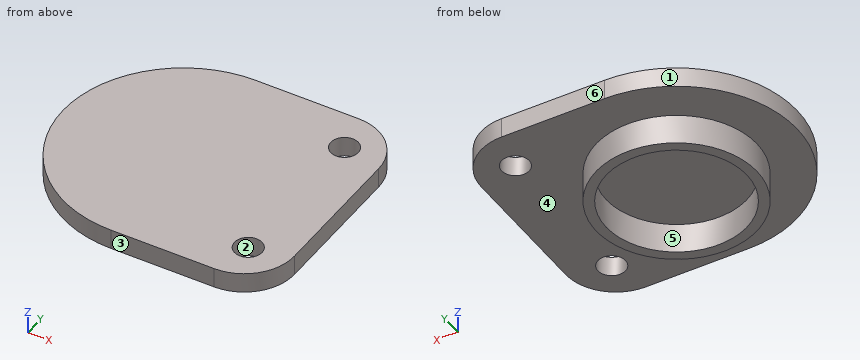
from build123d import *

# Parameters (mm, degrees)
SKETCH1_R           = 2.75
BOSS_EXTRUDE1_DEPTH = 4
SKETCH2_R           = 16
SKETCH2_R_2         = 14
BOSS_EXTRUDE2_DEPTH = 6


with BuildPart() as part:
    # Sketch1 → Boss-Extrude1 (new body)
    with BuildSketch(Plane.XY):
        with BuildLine():
            Line((0, -24), (20.5, -24))
            ThreePointArc((20.5, -24), (27.571067812, -21.071067812), (30.5, -14))
            Line((30.5, -14), (30.5, 14))
            ThreePointArc((30.5, 14), (27.571067812, 21.071067812), (20.5, 24))
            Line((20.5, 24), (0, 24))
            ThreePointArc((0, 24), (-24, 0), (0, -24))
        make_face()
        with Locations((22.5, -16)):
            Circle(SKETCH1_R, mode=Mode.SUBTRACT)
        with Locations((22.5, 16)):
            Circle(SKETCH1_R, mode=Mode.SUBTRACT)
    extrude(amount=BOSS_EXTRUDE1_DEPTH)

    # Sketch2 → Boss-Extrude2 (add)
    with BuildSketch(Plane(origin=(0, 0, 0), x_dir=(-1, 0, 0), z_dir=(0, 0, -1))):
        Circle(SKETCH2_R)
        Circle(SKETCH2_R_2, mode=Mode.SUBTRACT)
    extrude(amount=BOSS_EXTRUDE2_DEPTH)


solid = part.part
The listing builds one solid part. Answer for the finished solid, in the listing's coordinates (mm). Face numbers are marked on the shaded views. A direction names the side the tool comes from. Give positions to 0.01 mm unless a question says otherwise; leave off trailing zeros. Write each loop counter-clockwise with the first axis right and the second up, starting at its lowest first coordinate (ties: lowest second). Pieces come first, ordered by that corner, then holes. Notation, with made-up numbers: (-2, 29.25) -> (45, 29.25) arc R25 cw to (45, 44.25) -> close; hole circle Ø10 at (-7, 57). An arc over 180 degrees is marked (long way). One line per question, with ' | ' between items. Start each with the question number.
1. For a pull along Y with two mould halves and no side action, classify the marked faces 1, 2, 3 and 4 as pulls with the +Y half, pulls with the -Y half, needs draft (parallel to the pull), parting line crosses it, or undercut.
2. Section D-D (y = 0) is taken. Determine the outline of the cut face in (x, z).
3. Section B-B (x = 22.5) is taken. Determine the outline of the cut face in (y, z), plus the area to 3 significant figures.
4. Given pin 1 Ø5 at (y, z) = (-8, -4) entering from -X (3 decimals); pin 2 Ø6 at (x, z) = (-13.5, 1.5) entering from -Y; pin 3 Ø2 at (x, y) = (-17.5, 1) entering from -Z; pin 4 Ø1.5 at (x, z) = (5.5, -0.5) entering from +Y, each flat-ended and moving along its own axis, determine where each tip first touches the part or whether it passes through.
5. Section A-A (z = 0.75) is taken. Determine the outline of the cut face in (x, y), plus the area to 3 significant figures.
6. Find the intervals of material crossed by probe 1 along Y at (x, z) = (22.5, 1.35); probe 2 along Y at (x, z) = (0, -1.4); probe 3 along Z at (x, y) = (-0.5, 12.5), in increasing order.
7. Section C-C (y = -12) is taken. Determine the outline of the cut face in (x, z).
8. For the marked faces 5 and 6, determine the directions among +Z, -Z, +X, -X, +Y, -Y from which every point of the face is accessible in a straight line to the end or side of a thin tool.
Response values:
1) face 1: parting line crosses it | face 2: undercut | face 3: pulls with the -Y half | face 4: needs draft
2) outline: (-24, 0) -> (-16, 0) -> (-16, -6) -> (-14, -6) -> (-14, 0) -> (14, 0) -> (14, -6) -> (16, -6) -> (16, 0) -> (30.5, 0) -> (30.5, 4) -> (-24, 4) -> close
3) outline: (-23.8, 0) -> (-18.75, 0) -> (-18.75, 4) -> (-23.8, 4) -> close; (-13.25, 0) -> (13.25, 0) -> (13.25, 4) -> (-13.25, 4) -> close; (18.75, 0) -> (23.8, 0) -> (23.8, 4) -> (18.75, 4) -> close | area: 146 mm2
4) pin 1: x = -15.025 | pin 2: y = -21.58 | pin 3: z = 0 | pin 4: y = 24
5) outline: (0, -24) -> (20.5, -24) arc R10 ccw to (30.5, -14) -> (30.5, 14) arc R10 ccw to (20.5, 24) -> (0, 24) arc R24 ccw to start; hole circle Ø5.5 at (22.5, -16); hole circle Ø5.5 at (22.5, 16) | area: 2,280 mm2
6) probe 1: -23.8 to -18.75, -13.25 to 13.25, 18.75 to 23.8 | probe 2: -16 to -14, 14 to 16 | probe 3: 0 to 4
7) outline: (-20.78, 0) -> (-10.58, 0) -> (-10.58, -6) -> (-7.21, -6) -> (-7.21, 0) -> (7.21, 0) -> (7.21, -6) -> (10.58, -6) -> (10.58, 0) -> (30.5, 0) -> (30.5, 4) -> (-20.78, 4) -> close
8) face 5: -Z | face 6: +Z, -Z, +X, -X, +Y
